Design review of the part built by this model. Coordinates are the model's own, in mm. A direction names the side the tool comes from. Give positions to 0.01 mm unless a question says otherwise; leave off trailing zeros. Loops run counter-clockwise (first coordinate to the right, second up) from the corner with the lowest first, then second, coordinate; pieces in that order, holes last. Notation, with made-up numbers: (-7, 43.5) -> (29, 43.5) arc R33 ccw to (29, 75.5) -> close; hole circle Ø7 at (21, -15.75). An arc over 180 degrees is marked (long way). Answer as CSV lines item,"result".
Autodesk Inventor part; units mm, degrees
ref_plane "XY Plane" through (0, 0, 0) normal (0, 0, 1) x (1, 0, 0)
sketch "Sketch1" plane through (0, 0, 0) normal (1, 0, 0) x (0, 1, 0)
  circle A0 centre (0, 0) radius 2
  dimension "d0" = 4
extrude "Extrusion1" add sketch "Sketch1" along normal blind 28.5
sketch "Sketch2" plane through (28.5, 0, 0) normal (1, 0, 0) x (0, 0, -1)
  circle A0 centre (0, 0) radius 1.5
  dimension "d3" = 3
extrude "Extrusion2" cut sketch "Sketch2" against normal blind 0.25
sketch "Sketch3" plane through (28.25, 0, 0) normal (1, 0, 0) x (0, 0, -1)
  circle A0 centre (0, 0) radius 1.25
  dimension "d6" = 2.5
extrude "Extrusion3" cut sketch "Sketch3" against normal blind 5.75
sketch "Sketch4" plane through (0, 0, 0) normal (-1, 0, 0) x (0, 0, 1)
  circle A0 centre (0, 0) radius 3.5
  dimension "d9" = 7
extrude "Extrusion4" add sketch "Sketch4" along normal blind 22.5
ref_plane "Work Plane1" through (-17.5, 0, 0) normal (-1, 0, 0) x (0, 0, 1)
sketch "Sketch5" plane through (-17.5, 0, 0) normal (-1, 0, 0) x (0, 0, 1)
  circle A0 centre (0, 0) radius 3
  circle A1 centre (0, 0) radius 3.5
  dimension "d13" = 6
  dimension "d14" = 7
extrude "Extrusion5" cut sketch "Sketch5" against normal blind 1
ref_plane "Work Plane2" through (-14, 0, 0) normal (-1, 0, 0) x (0, 0, 1)
sketch "Sketch7" plane through (-14, 0, 0) normal (-1, 0, 0) x (0, 0, 1)
  circle A0 centre (0, 0) radius 3
  circle A1 centre (0, 0) radius 3.5
  dimension "d18" = 7
  dimension "d19" = 6
extrude "Extrusion6" cut sketch "Sketch7" against normal blind 1
ref_plane "Work Plane3" through (-10.5, 0, 0) normal (-1, 0, 0) x (0, 0, 1)
sketch "Sketch9" plane through (-10.5, 0, 0) normal (-1, 0, 0) x (0, 0, 1)
  circle A0 centre (0, 0) radius 3
  circle A1 centre (0, 0) radius 3.5
  dimension "d25" = 7
  dimension "d26" = 6
extrude "Extrusion7" cut sketch "Sketch9" against normal blind 1
ref_plane "Work Plane4" through (-7, 0, 0) normal (-1, 0, 0) x (0, 0, 1)
sketch "Sketch10" plane through (-7, 0, 0) normal (-1, 0, 0) x (0, 0, 1)
  circle A0 centre (0, 0) radius 3
  circle A1 centre (0, 0) radius 3.5
  dimension "d30" = 7
  dimension "d31" = 6
extrude "Extrusion8" cut sketch "Sketch10" against normal blind 1
ref_plane "Work Plane5" through (-3.5, 0, 0) normal (-1, 0, 0) x (0, 0, 1)
sketch "Sketch11" plane through (-3.5, 0, 0) normal (-1, 0, 0) x (0, 0, 1)
  circle A0 centre (0, 0) radius 2
  circle A1 centre (0, 0) radius 3
  circle A2 centre (0, 0) radius 3.5
  dimension "d35" = 7
  dimension "d36" = 6
extrude "Extrusion9" cut sketch "Sketch11" against normal blind 1 contours A2
Q1. We need section A-A, the plane x = 25.5. State the section outline as (y, z) points.
Filled sheet:
outline,"circle Ø4 at (0, 0); hole circle Ø2.5 at (0, 0)"
Q2. We need section B-B, the plane x = 7.5. State the section outline as (y, z) points.
Filled sheet:
outline,"circle Ø4 at (0, 0)"
Q3. To check wall thickness, follow probe 1 along X at (y, z) = (2, 2.75); probe 2 along X at (y, z) = (0.5, -2); probe 3 along Y at (x, z) = (6, 0.25). State the ranges of each line that lie inside material, in increasing order. Write a range as from..to.
Filled sheet:
probe 1,"x = -22.5..-17.5, -16.5..-14, -13..-10.5, -9.5..-7, -6..-3.5, -2.5..0"
probe 2,"x = -22.5..0"
probe 3,"y = -1.98..1.98"
Q4. For faces 1 (the cylindrical face through (-15.232, 1.341, 3.233)), 2 (the cylindrical face through (25.42, -1.22, 0.27)), 3 (the cylindrical face through (-13.5, 0.1, -3)), list the 3-axis set-ups (+Z, -Z, +X, -X, +Y, -Y) from which the entire face can be reached by the end or side of a thin tool; tool diameter is ignored.
Filled sheet:
face 1,"+X, -X"
face 2,"+X"
face 3,"none"
Q5. Clearance check with flat-ended pins moving along their axes: pin 1 Ø4 at (x, z) = (19.5, -0.5) entering from +Y; pin 2 Ø1.5 at (x, z) = (-17, -1.5) entering from -Y; pin 3 Ø3.5 at (y, z) = (0, -0.5) entering from +X; pin 4 Ø3 at (x, y) = (17.5, 2.5) entering from +Z. State where each tip first meets the part, or that it passes through.
Filled sheet:
pin 1,"stops at y = 2"
pin 2,"stops at y = -3.37"
pin 3,"stops at x = 28.5"
pin 4,"stops at z = 1.73"
Q6. The part is to be moulded in two halves that separate along X. For faces 4 (the cylindrical face through (-1.232, 1.341, 3.233)), 5 (the cylindrical face through (-6.5, 0.1, -3)), 6 (the flat face through (0, -2, 2)), say which applies: pulls with the +X half, pulls with the -X half, needs draft (parallel to the pull), parting line crosses it, or undercut.
Filled sheet:
face 4,"needs draft"
face 5,"undercut"
face 6,"pulls with the +X half"
